Part model, mm, in its own coordinate system. A direction names the side the tool comes from. Round coordinates to 2 decimals unless told otherwise and drop trailing zeros. Loops run counter-clockwise (first coordinate to the right, second up) from the corner with the lowest first, then second, coordinate; pieces in that order, holes last.
1) Probe line 1 (X direction, y = -4.5, z = -12) (3 decimals); line 2 (Z direction, x = -2.25, y = -0.25); line 3 (Y direction, x = 0, z = -18.25). List the from-to ranges inside material, lowest first.
2) Band-saw the part on D-D, the plane y = -1.5. Write the cut outline in (x, z) (3 decimals).
3) Band-saw the part on A-A, the plane y = 0. Write the cut outline in (x, z) (3 decimals), then the cut area to 3 significant figures.
4) Band-saw the part on C-C, the plane z = -17. Write the cut outline in (x, y) (3 decimals), then the cut area to 3 significant figures.
5) Mould opens along Z. For faces 4 (the flat face through (3.175, 0, -10)), 5 (the cylindrical face through (-0.044, 0.954, -12.847)), 6 (the flat face through (0, 0, 0)), 7 (the flat face through (-4, 0, -3.175)) say: +Z half, -Z half, draft (parallel to the pull), parting line (faces both ways), or undercut.
6) 3-axis set-ups, long thin cutter, end or side, ignore diameter. For faces 1 (the flat face through (-3.175, 0, -10)), 2 (the flat face through (4, 0, -3.175)), 3 (the cylindrical face through (-2.93, 5.634, -6.062)): which of +Z, -Z, +X, -X, +Y, -Y reach the whole face in a straight line?
7) Drop flat-ended pins along their axis: P1, Ø6, axis at y = -1.5, z = -9.5, coming from the -X side (3 decimals); P2, Ø4, axis at x = -2.5, z = -19, coming from the -Y side; P3, Ø1.6, axis at x = -4.5, y = -1.5, coming from the -Z side (3 decimals); P4, Ø5.5, axis at y = 0, z = -15.875, coming from the -X side. Give the stop position or say it passes through.
8) Band-saw the part on B-B, the plane x = 0. Write the cut outline in (y, z) (3 decimals), then the cut area to 3 significant figures.
from build123d import *

# Parameters (mm, degrees)
SKETCH2_W          = 12.7
SKETCH2_H          = 60.004179461
CUT_EXTRUDE1_DEPTH = 24.970724332
SKETCH3_R          = 3.175
CUT_EXTRUDE2_DEPTH = 25.999975


with BuildPart() as part:
    # Sketch1 → Revolve1 (revolve)
    with BuildSketch(Plane(origin=(0, 0, 0), x_dir=(1, 0, 0), z_dir=(0, 1, 0)), mode=Mode.PRIVATE) as revolve1_sk:
        with BuildLine():
            Line((0, 0), (0, 15.875))
            Line((0, 15.875), (0, 22.225))
            ThreePointArc((0, 22.225), (4.490128061, 20.365128061), (6.35, 15.875))
            Line((6.35, 15.875), (6.35, 0))
            Line((6.35, 0), (0, 0))
        make_face()
    revolve(revolve1_sk.sketch.rotate(Axis((0, 0, -22.225), (0, 0, 1)), 180), axis=Axis((0, 0, -22.225), (0, 0, 1)))

    # Sketch2 → Cut-Extrude1 (cut, symmetric)
    with BuildSketch(Plane(origin=(0, 0, 0), x_dir=(1, 0, 0), z_dir=(0, 1, 0))):
        with Locations((-9.525, 33.177089731)):
            Rectangle(SKETCH2_W, SKETCH2_H)
    cut_extrude1 = extrude(amount=CUT_EXTRUDE1_DEPTH, both=True, mode=Mode.SUBTRACT)

    # Mirror1: Cut-Extrude1 across plane
    add(cut_extrude1.mirror(Plane(origin=(0, 0, 0), x_dir=(0, 0, 1), z_dir=(1, 0, 0))), mode=Mode.SUBTRACT)

    # Sketch3 → Cut-Extrude2 (cut, through all)
    with BuildSketch(Plane.ZY.offset(3.175)):
        with Locations((-15.875, 0)):
            Circle(SKETCH3_R)
    extrude(amount=-CUT_EXTRUDE2_DEPTH, mode=Mode.SUBTRACT)


solid = part.part
Reported:
1. line 1: x = -3.175 to 3.175
1. line 2: z = -21.81 to -19.04, -12.71 to 0
1. line 3: y = -5.89 to -2.11, 2.11 to 5.89
2. outline: (-6.17, -3.175) - (-3.175, -3.175) - (-3.175, -13.077) - (3.175, -13.077) - (3.175, -3.175) - (6.17, -3.175) - (6.17, 0) - (-6.17, 0) - close; (-3.175, -21.166) arc R6.17 ccw to (3.175, -21.166) - (3.175, -18.673) - (-3.175, -18.673) - close
3. outline: (-6.35, -3.175) - (-3.175, -3.175) - (-3.175, -12.7) - (3.175, -12.7) - (3.175, -3.175) - (6.35, -3.175) - (6.35, 0) - (-6.35, 0) - close; (-3.175, -21.374) arc R6.35 ccw to (3.175, -21.374) - (3.175, -19.05) - (-3.175, -19.05) - close
3. area: 119 mm2
4. outline: (-3.175, -5.383) arc R6.25 ccw to (3.175, -5.383) - (3.175, -2.969) - (-3.175, -2.969) - close; (-3.175, 2.969) - (3.175, 2.969) - (3.175, 5.383) arc R6.25 ccw to (-3.175, 5.383) - close
4. area: 38.1 mm2
5. face 4: draft
5. face 5: undercut
5. face 6: +Z half
5. face 7: -Z half
6. face 1: -Z, -X, +Y, -Y
6. face 2: -Z, +X, +Y, -Y
6. face 3: +Z, -Z
7. P1: stops at x = -3.175
7. P2: stops at y = -6.03
7. P3: stops at z = -3.175
7. P4: passes through
8. outline: (-6.35, -15.875) arc R6.35 ccw to (6.35, -15.875) - (6.35, 0) - (-6.35, 0) - close; hole circle Ø6.35 at (0, -15.875)
8. area: 233 mm2
